from build123d import *

# Parameters (mm, degrees)
ESQUISSE1_W             = 20.5
ESQUISSE1_H             = 20.5
BOSS_EXTRU_1_DEPTH      = 32
ESQUISSE2_W             = 20.5
ESQUISSE2_H             = 20.5
ESQUISSE2_R             = 8
ESQUISSE2_R_2           = 1.25
BOSS_EXTRU_2_DEPTH      = 2
ESQUISSE4_W             = 12
ESQUISSE4_H             = 2
ENL_V_MAT_EXTRU_2_DEPTH = 10
CONG_1_R                = 1
ENL_V_MAT_EXTRU_3_REACH = 38.5
ESQUISSE5_R             = 2.1


with BuildPart() as part:
    # Esquisse1 → Boss.-Extru.1 (new body)
    with BuildSketch(Plane(origin=(0, 0, 0), x_dir=(1, 0, 0), z_dir=(0, 1, 0))):
        Polygon((0, 0), (24.5, 0), (24.5, 34.5), (34.5, 34.5), (34.5, 36.5), (24.5, 36.5), (0, 36.5), (-10, 36.5), (-10, 34.5), (0, 34.5), align=None)
        with Locations((12.25, 12.25)):
            Rectangle(ESQUISSE1_W, ESQUISSE1_H, mode=Mode.SUBTRACT)
    extrude(amount=BOSS_EXTRU_1_DEPTH)

    # Esquisse2 → Boss.-Extru.2 (add)
    with BuildSketch(Plane.XZ):
        with Locations((12.25, -12.25)):
            Rectangle(ESQUISSE2_W, ESQUISSE2_H)
        with Locations((12.25, -12.25)):
            Circle(ESQUISSE2_R, mode=Mode.SUBTRACT)
        with Locations((3.5, -3.5)):
            Circle(ESQUISSE2_R_2, mode=Mode.SUBTRACT)
        with Locations((21, -3.5)):
            Circle(ESQUISSE2_R_2, mode=Mode.SUBTRACT)
        with Locations((21, -21)):
            Circle(ESQUISSE2_R_2, mode=Mode.SUBTRACT)
        with Locations((3.5, -21)):
            Circle(ESQUISSE2_R_2, mode=Mode.SUBTRACT)
    extrude(amount=-BOSS_EXTRU_2_DEPTH)

    # Esquisse4 → Enlèv. mat.-Extru.2 (cut)
    with BuildSketch(Plane(origin=(0, 32, 0), x_dir=(1, 0, 0), z_dir=(0, 1, 0))):
        with Locations((12.25, 1)):
            Rectangle(ESQUISSE4_W, ESQUISSE4_H)
    extrude(amount=-ENL_V_MAT_EXTRU_2_DEPTH, mode=Mode.SUBTRACT)

    # Congé1
    cong_1_edges = [part.edges().sort_by_distance(p)[0] for p in [
        (2, 32, -12.25),
        (4.125, 32, -2),
        (22.5, 32, -12.25),
        (12.25, 32, -22.5),
        (20.375, 32, -2),
        (12.25, 22, -2),
        (6.25, 27, -2),
        (18.25, 27, -2),
        (6.25, 32, -1),
        (18.25, 32, -1),
    ]]
    fillet(cong_1_edges, radius=CONG_1_R)

    # Esquisse5 → Enlèv. mat.-Extru.3 (cut, up to next)
    with BuildSketch(Plane(origin=(0, 0, -36.5), x_dir=(-1, 0, 0), z_dir=(0, 0, -1)), mode=Mode.PRIVATE) as enl_v_mat_extru_3_sk1:
        with Locations((-29.5, 5)):
            Circle(ESQUISSE5_R)
    enl_v_mat_extru_3_tool1 = extrude(enl_v_mat_extru_3_sk1.sketch, amount=-ENL_V_MAT_EXTRU_3_REACH, mode=Mode.PRIVATE) & part.part
    add(enl_v_mat_extru_3_tool1.solids().sort_by_distance((29.5, 5, -36.5))[0], mode=Mode.SUBTRACT)
    # Esquisse5 → Enlèv. mat.-Extru.3 (cut, up to next)
    with BuildSketch(Plane(origin=(0, 0, -36.5), x_dir=(-1, 0, 0), z_dir=(0, 0, -1)), mode=Mode.PRIVATE) as enl_v_mat_extru_3_sk2:
        with Locations((5, 5)):
            Circle(ESQUISSE5_R)
    enl_v_mat_extru_3_tool2 = extrude(enl_v_mat_extru_3_sk2.sketch, amount=-ENL_V_MAT_EXTRU_3_REACH, mode=Mode.PRIVATE) & part.part
    add(enl_v_mat_extru_3_tool2.solids().sort_by_distance((-5, 5, -36.5))[0], mode=Mode.SUBTRACT)


solid = part.part
Verification items for the finished model (mm, model axes). A direction names the side the tool comes from. Coordinates: 2 decimals unless noted, no trailing zeros. Write each loop counter-clockwise with the first axis right and the second up, starting at its lowest first coordinate (ties: lowest second). Pieces come first, ordered by that corner, then holes. Notation, with made-up numbers: (31, -27.75) -> (55, -27.75) arc R12 ccw to (55, -17.75) -> close; hole circle Ø5 at (85, -33). An arc over 180 degrees is marked (long way). One line per item, written item: value. Start each with the question number.
Q1. Go/stop test with flat-tipped pins: P1, Ø3, axis at x = 19.5, z = -19.5, coming from the +Y side; P2, Ø12, axis at y = 23, z = -7.5, coming from the -X side; P3, Ø1.5, axis at x = 3.5, z = -3.5, coming from the -Y side; P4, Ø21, axis at x = 12.25, z = -12.25, coming from the +Y side. Record where each tip stops, or that it passes through.
Q2. Cross-section at D-D on z = -21. Enter the section's corners in (x, y), and give its area (3 significant figures).
Q3. Thickness scan on L1, parallel to Z at x = 3.5, y = 1.6; L2, parallel to Z at x = 18, y = 19.5; L3, parallel to X at y = 11, z = -4.5. Record the ranges inside material, lowest first. Write a range as from..to.
Q4. Access from +Z, -Z, +X, -X, +Y, -Y to the whole of each face (thin tool, end or side, straight path). Record for faces 4 (the flat face through (-5, 16, -34.5)), 5 (the cylindrical face through (4.655, 0.986, -3.979)), 6 (the cylindrical face through (5.949, 31.715, -0.507)), 7 (the flat face through (12, 32, -28)), 8 (the cylindrical face through (22.785, 31.699, -12.408)).
Q5. Cross-section at B-B on z = -12.25. Enter the section's corners in (x, y), and give its area (3 significant figures).
Q6. Cross-section at A-A on x = -5. Enter the section's corners in (y, z), and give its area (3 significant figures).
Q7. Cross-section at C-C on x = 3.5. Enter the section's corners in (y, z).
Q8. Mould release check, pull along X, two halves, no side actions. Record for faces 1 (the flat face through (12, 12, 0)), 2 (the cylindrical face through (3.627, 31.699, -1.715)), 3 (the flat face through (24.5, 16, -17)): pulls with the +X half, pulls with the -X half, needs draft (parallel to the pull), parting line crosses it, or undercut.
Checked values:
1. P1: stops at y = 2
1. P2: stops at x = 0
1. P3: passes through
1. P4: stops at y = 31.66
2. outline: (0, 0) -> (2.25, 0) -> (2.25, 2) -> (2, 2) -> (2, 31) arc R1 ccw to (1, 32) -> (0, 32) -> close; (4.75, 0) -> (19.75, 0) -> (19.75, 2) -> (4.75, 2) -> close; (22.25, 0) -> (24.5, 0) -> (24.5, 32) -> (23.5, 32) arc R1 ccw to (22.5, 31) -> (22.5, 2) -> (22.25, 2) -> close
2. area: 159 mm²
3. L1: z = -36.5..-22.25, -19.75..-4.75, -2.25..0
3. L2: z = -36.5..-22.5, -2..0
3. L3: x = 0..2, 22.5..24.5
4. face 4: +Z, -X, +Y, -Y
4. face 5: +Y, -Y
4. face 6: +Z, +Y
4. face 7: +Z, -Z, +X, -X, +Y
4. face 8: +Y
5. outline: (0, 0) -> (4.25, 0) -> (4.25, 2) -> (2, 2) -> (2, 31) arc R1 ccw to (1, 32) -> (0, 32) -> close; (20.25, 0) -> (24.5, 0) -> (24.5, 32) -> (23.5, 32) arc R1 ccw to (22.5, 31) -> (22.5, 2) -> (20.25, 2) -> close
5. area: 137 mm²
6. outline: (0, -36.5) -> (2.9, -36.5) -> (2.9, -34.5) -> (0, -34.5) -> close; (7.1, -36.5) -> (32, -36.5) -> (32, -34.5) -> (7.1, -34.5) -> close
6. area: 55.6 mm²
7. outline: (0, -36.5) -> (32, -36.5) -> (32, -23.5) arc R1 ccw to (31, -22.5) -> (2, -22.5) -> (2, -22.25) -> (0, -22.25) -> close; (0, -19.75) -> (2, -19.75) -> (2, -4.75) -> (0, -4.75) -> close; (0, -2.25) -> (2, -2.25) -> (2, -2) -> (31, -2) arc R1 ccw to (32, -1) -> (32, 0) -> (0, 0) -> close
8. face 1: needs draft
8. face 2: undercut
8. face 3: pulls with the +X half
